Part model, mm, in its own coordinate system. Face numbers are marked on the shaded views. A direction names the side the tool comes from. Give positions to 0.01 mm unless a question says otherwise; leave off trailing zeros. Write each loop counter-clockwise with the first axis right and the second up, starting at its lowest first coordinate (ties: lowest second). Pieces come first, ordered by that corner, then holes. Notation, with made-up numbers: (-15.5, 12) - (17.5, 12) arc R10 ccw to (17.5, 18) - close; hole circle Ø5 at (45, -38.5). An arc over 180 degrees is marked (long way). Answer as a JSON object with one key per item and string values. Group by question number.
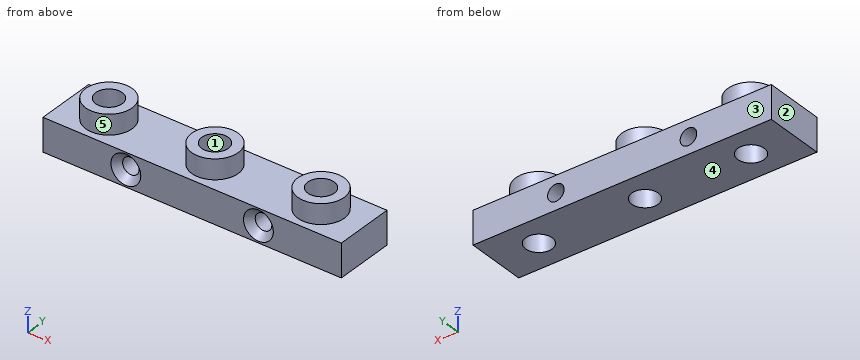
Autodesk Fusion 360 part; units mm, degrees
sketch "Sketch1" plane through (0, 0, 0) normal (0, 0, 1) x (1, 0, 0)
  line L0 (0, 0) -> (90, 0)
  line L1 (90, 0) -> (90, 18)
  line L2 (90, 18) -> (0, 18)
  line L3 (0, 18) -> (0, 0)
  circle A0 centre (13, 9) radius 4
  circle A1 centre (45, 9) radius 4
  circle A2 centre (77, 9) radius 4
  circle A3 centre (13, 9) radius 7
  circle A4 centre (45, 9) radius 7
  circle A5 centre (77, 9) radius 7
  dimension "d1" = 9
  dimension "d2" = 9
  dimension "d3" = 9
  dimension "d4" = 45
  dimension "d5" = 32
  dimension "d6" = 32
extrude "Extrude1" add sketch "Sketch1" along normal blind 10 contours L0 L1 L2 L3 | A3 | A4 | A5
extrude "Extrude2" add sketch "Sketch1" along normal blind 16 contours A3 | A4 | A5
sketch "Sketch2" plane through (0, 0, 0) normal (0, -1, 0) x (1, 0, 0)
  line L0 (0, 0) -> (90, 0)
  line L1 (90, 0) -> (90, 10)
  line L2 (90, 10) -> (0, 10)
  line L3 (0, 10) -> (0, 0)
  circle A0 centre (25, 5) radius 2.5
  circle A1 centre (65, 5) radius 2.5
  dimension "d11" = 25
  dimension "d12" = 40
extrude "Extrude3" cut sketch "Sketch2" against normal blind 18 contours A0 | A1
chamfer "Chamfer1" distance 2 angle 45 2 edges at (62.6692, 0, 5.904) (22.6692, 0, 5.904)
1) Saw through at B-B (z = 5). List the corners of the cut face in (x, y).
2) Two-plate mould, pull along X, no slides. Class the marked faces 1, 2 and 3: +X half, -X half, draft (parallel to the pull), parting line (faces both ways), or undercut.
3) Which spindle directions (+Z, -Z, +X, -X, +Y, -Y) get a long thin tool onto all of the face, cutting with end or side? Do the marked faces 4 and 5. Say none if no direction does.
4) Saw through at C-C (x = 65). List the corners of the cut face in (y, z).
5) Drop flat-ended pins along their axis: P1, Ø6.5, axis at x = 77, y = 9, coming from the -Z side; P2, Ø1, axis at x = 48, z = 13.5, coming from the +Y side. Give the stop position or say it passes through.
6) Saw through at A-A (y = 9). State how many separate pieces and enclosed holes the cut face has, and give its area (3 significant figures).
7) Drill centre lines: line 1 along X through (y, z) = (8.75, 7.75); line 2 along X through (y, z) = (4.25, 15); line 3 along Y through (x, z) = (77, 11). Where is each one in solid material? Low to high. Write a range as from..to.
8) Saw through at D-D (y = 13.75). List the corners of the cut face in (x, z).
Checks:
{
 "1": {"outline": "(0, 0) - (20.5, 0) - (22.5, 2) - (22.5, 18) - (0, 18) - close; (27.5, 2) - (29.5, 0) - (60.5, 0) - (62.5, 2) - (62.5, 18) - (27.5, 18) - close; (67.5, 2) - (69.5, 0) - (90, 0) - (90, 18) - (67.5, 18) - close; hole circle Ø8 at (13, 9); hole circle Ø8 at (45, 9); hole circle Ø8 at (77, 9)"},
 "2": {"face 1": "undercut", "face 2": "-X half", "face 3": "draft"},
 "3": {"face 4": "-Z, +X, -X, +Y, -Y", "face 5": "+Z"},
 "4": {"outline": "(0, 0) - (18, 0) - (18, 2.5) - (2, 2.5) - (0, 0.5) - close; (0, 9.5) - (2, 7.5) - (18, 7.5) - (18, 10) - (0, 10) - close"},
 "5": {"P1": "through", "P2": "y = 15.54"},
 "6": {"separate pieces": "4", "enclosed holes": "2", "area": "729 mm2"},
 "7": {"line 1": "0..9.01, 16.99..41.01, 48.99..73.01, 80.99..90", "line 2": "7.86..18.14, 39.86..50.14, 71.86..82.14", "line 3": "2..5, 13..16"},
 "8": {"outline": "(0, 0) - (90, 0) - (90, 10) - (82.14, 10) - (82.14, 16) - (71.86, 16) - (71.86, 10) - (50.14, 10) - (50.14, 16) - (39.86, 16) - (39.86, 10) - (18.14, 10) - (18.14, 16) - (7.86, 16) - (7.86, 10) - (0, 10) - close; hole circle Ø5 at (25, 5); hole circle Ø5 at (65, 5)"}
}
